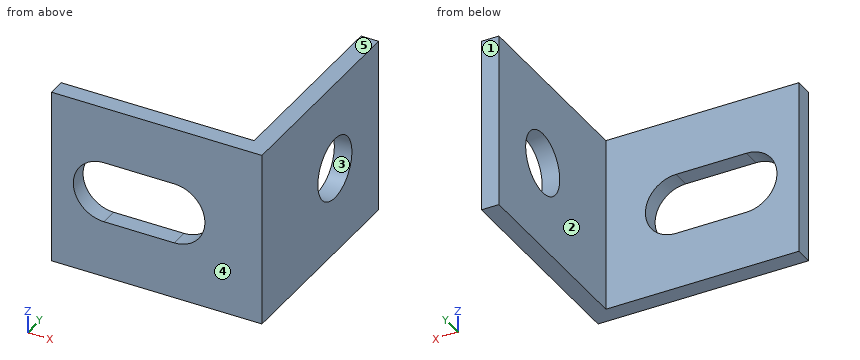
from build123d import *

# Parameters (mm, degrees)
F1_DEPTH = 10
F4_D     = 3.5
F5_DEPTH = 25


with BuildPart() as f1:
    # F0 (on Top) → F1 (new body)
    with BuildSketch(Plane.XY):
        Polygon((-12, 0), (0, 0), (0, 12), (-1, 12), (-1, 1), (-12, 1), align=None)
    extrude(amount=F1_DEPTH)

    # F4 (through all)
    with Locations(Plane(origin=(-1, 0, 0), x_dir=(0, -1, 0), z_dir=(-1, 0, 0))):
        with Locations((-7.5, 5)):
            Hole(F4_D / 2)

    # F2 (on face) → F5 (cut)
    with BuildSketch(Plane(origin=(0, 1, 0), x_dir=(-1, 0, 0), z_dir=(0, 1, 0))):
        with BuildLine():
            Line((9, 6.75), (5, 6.75))
            ThreePointArc((5, 6.75), (3.25, 5), (5, 3.25))
            Line((5, 3.25), (9, 3.25))
            ThreePointArc((9, 3.25), (10.75, 5), (9, 6.75))
        make_face()
    extrude(amount=-F5_DEPTH, mode=Mode.SUBTRACT)


solid = f1.part
The model under review builds one solid part; all positions refer to its coordinate system, in mm. Face numbers are marked on the shaded views. A direction names the side the tool comes from. Coordinates: 2 decimals unless noted, no trailing zeros. Loops run counter-clockwise (first coordinate to the right, second up) from the corner with the lowest first, then second, coordinate; pieces in that order, holes last. Notation, with made-up numbers: M -32,35 L -23,35 A28 cw -23,65 Z; hole C 73.5,-14.75 d7. An arc over 180 degrees is marked long. Put each result on its own line as item: value. Start each with the question number.
Q1. Add section B-B (y = 7.5). Write out the cut boundary in (x, z).
Q2. Clearance check with flat-ended pins moving along their axes: pin 1 (6 mm diameter, centred on y = 7.5, z = 6.5, fed in from -X); pin 2 (1 mm diameter, centred on x = -3.5, z = 2.5, fed in from +Y); pin 3 (4 mm diameter, centred on x = -1.5, y = 2, fed in from +Z). State where each tip first meets the part, or that it passes through.
Q3. Add section A-A (x = -6.75). Write out the cut boundary in (y, z), and give its area (3 significant figures).
Q4. Wall thickness on line 1 (Z direction, x = -0.65, y = 7.5); line 2 (Y direction, x = -2.75, z = 3.5); line 3 (X direction, y = 5.5, z = 5.5): over which ranges is each line inside the solid? List them lowest first.
Q5. The part is to be moulded in two halves that separate along Y. For the marked faces 3, 4 and 5, say which applies: +Y half, -Y half, draft (parallel to the pull), parting line (faces both ways), or undercut.
Q6. For the marked faces 1 and 2, list the 3-axis set-ups (+Z, -Z, +X, -X, +Y, -Y) from which the entire face can be reached by the end or side of a thin tool; tool diameter is ignored.
Q7. Add section C-C (z = 5). Write out the cut boundary in (x, y), and give its area (3 significant figures).
Q8. Add section D-D (z = 6.25). Write out the cut boundary in (x, y).
Answers:
1. outline: M -1,0 L 0,0 L 0,3.25 L -1,3.25 Z; M -1,6.75 L 0,6.75 L 0,10 L -1,10 Z
2. pin 1: stops at x = -1
2. pin 2: stops at y = 1
2. pin 3: stops at z = 10
3. outline: M 0,0 L 1,0 L 1,3.25 L 0,3.25 Z; M 0,6.75 L 1,6.75 L 1,10 L 0,10 Z
3. area: 6.50 mm^2
4. line 1: z = 0 to 3.25, 6.75 to 10
4. line 2: y = 0 to 1
4. line 3: x = -1 to 0
5. face 3: undercut
5. face 4: -Y half
5. face 5: draft
6. face 1: +Z, -Z, +X, -X, +Y
6. face 2: +Z, -Z, -X, +Y
7. outline: M -12,0 L -10.75,0 L -10.75,1 L -12,1 Z; M -3.25,0 L 0,0 L 0,5.75 L -1,5.75 L -1,1 L -3.25,1 Z; M -1,9.25 L 0,9.25 L 0,12 L -1,12 Z
7. area: 12.0 mm^2
8. outline: M -12,0 L -10.22,0 L -10.22,1 L -12,1 Z; M -3.78,0 L 0,0 L 0,6.28 L -1,6.28 L -1,1 L -3.78,1 Z; M -1,8.72 L 0,8.72 L 0,12 L -1,12 Z
